The figure shows three views and two pictorial views of one solid part (mm, origin at its lowest corner). Answer the questions. Give positions to 0.01 mm unless a question says otherwise; leave off trailing zeros. Loops run counter-clockwise (first coordinate to the right, second up) from the corner with the lowest first, then second, coordinate; pieces in that order, holes last. Notation, with made-up numbers: M 41,59 L 91,59 A25 ccw 91,92 Z; hole C 58,66.5 d5. An arc over 180 degrees is marked long. One line per item, written item: value. Start each with the question number.
Q1. Consider L1, parallel to X at y = 5.6, z = 35 (1 decimal); L2, parallel to X at y = 2.4, z = 32.5 (1 decimal); L3, parallel to Z at x = 18, y = 5.3 (1 decimal). Determine where each line is inside the solid, lowest interval first.
Q2. Flat-ended cylindrical pins translate along their axes: pin 1 (1.5 mm diameter, centred on x = 3, y = 3.5, fed in from -Z) (1 decimal); pin 2 (3 mm diameter, centred on x = 23, y = 3.5, fed in from +Z); pin 3 (2 mm diameter, centred on y = 2.5, z = 16, fed in from -X). Find the tip coordinate at first contact, or state that the pin passes through.
Q3. A cutting plane is placed at A-A, the plane z = 32.5. Determine the outline of the cut face in (x, y).
Q4. The mould has two halves that part along Z. Classify the marked faces 1, 2 and 3: +Z half, -Z half, draft (parallel to the pull), parting line (faces both ways), or undercut.
Q5. A cutting plane is placed at B-B, the plane x = 17.5. Determine the outline of the cut face in (y, z) (1 decimal).
Q6. A cutting plane is placed at D-D, the plane x = 5.5. Determine the outline of the cut face in (y, z) (1 decimal).
Q7. A cutting plane is placed at C-C, the plane y = 0.7. State how many separate pieces and enclosed holes the cut face has, and give its area (3 significant figures).
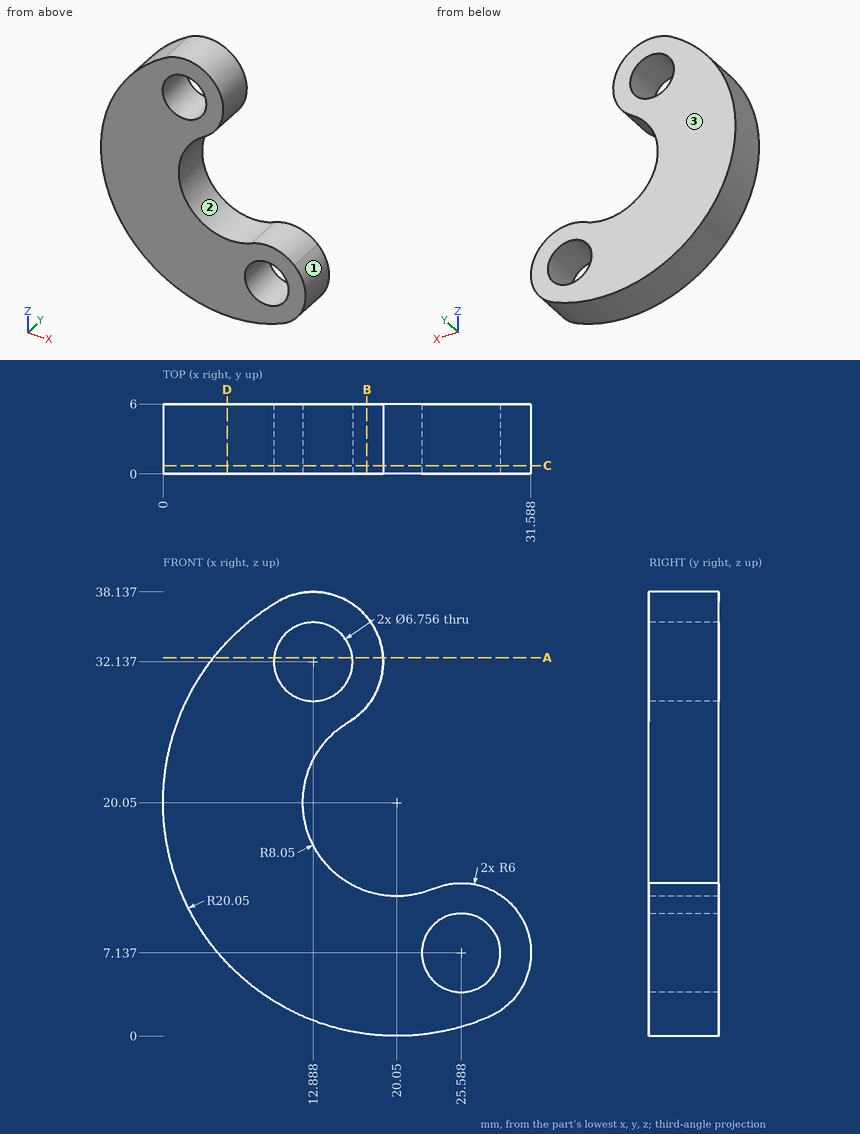
Answer block:
1. L1: 6.7 to 11.1, 14.7 to 18.2
1. L2: 4.3 to 9.5, 16.2 to 18.9
1. L3: 0.1 to 12.3, 29 to 35.3
2. pin 1: z = 8.4
2. pin 2: z = 13.04
2. pin 3: x = 0.23
3. outline: M 4.33,0 L 9.53,0 L 9.53,6 L 4.33,6 Z; M 16.25,0 L 18.88,0 L 18.88,6 L 16.25,6 Z
4. face 1: parting line
4. face 2: undercut
4. face 3: draft
5. outline: M 0,0.2 L 6,0.2 L 6,12.4 L 0,12.4 Z; M 0,28.3 L 6,28.3 L 6,36 L 0,36 Z
6. outline: M 0,6.3 L 6,6.3 L 6,33.8 L 0,33.8 Z
7. separate pieces: 1
7. enclosed holes: 2
7. area: 549 mm^2
